```python
from build123d import *

# Parameters (mm, degrees)
BOSS_EXTRUDE1_DEPTH = 56.75
SKETCH2_W           = 5
SKETCH2_H           = 85
SKETCH2_R           = 1.5875
CUT_EXTRUDE1_DEPTH  = 2
SKETCH3_R           = 6.35
SKETCH3_R_2         = 1.5875
CUT_EXTRUDE2_DEPTH  = 3
CHAMFER1_SIZE       = 0.5
CUT_EXTRUDE3_DEPTH  = 5.5
CUT_EXTRUDE4_DEPTH  = 10


with BuildPart() as part:
    # Sketch1 → Boss-Extrude1 (new body, symmetric)
    with BuildSketch(Plane.XY):
        Polygon((0, 50), (0, -50), (7.5, -50), (7.5, -42.5), (2, -42.5), (2, 42.5), (7.5, 42.5), (7.5, 50), align=None)
    extrude(amount=BOSS_EXTRUDE1_DEPTH, both=True)

    # Sketch2 → Cut-Extrude1 (cut)
    with BuildSketch(Plane(origin=(2, 0, 0), x_dir=(0, 0, -1), z_dir=(1, 0, 0))):
        with Locations((-54.25, 0)):
            Rectangle(SKETCH2_W, SKETCH2_H)
        with Locations((54.25, 0)):
            Rectangle(SKETCH2_W, SKETCH2_H)
        with Locations((-47.75, 17.5)):
            Circle(SKETCH2_R)
        with Locations((-47.75, -17.5)):
            Circle(SKETCH2_R)
        with Locations((47.75, 17.5)):
            Circle(SKETCH2_R)
        with Locations((47.75, -17.5)):
            Circle(SKETCH2_R)
    extrude(amount=-CUT_EXTRUDE1_DEPTH, mode=Mode.SUBTRACT)

    # Sketch3 → Cut-Extrude2 (cut, through all)
    with BuildSketch(Plane(origin=(2, 0, 0), x_dir=(0, 0, -1), z_dir=(1, 0, 0))):
        Circle(SKETCH3_R)
        with Locations((39.75, 30.5)):
            Circle(SKETCH3_R_2)
        with Locations((39.75, -30.5)):
            Circle(SKETCH3_R_2)
        with BuildLine():
            Line((-29.899655804, -39.5), (29.899655804, -39.5))
            ThreePointArc((29.899655804, -39.5), (32.863003185, -37.464823364), (32.027336169, -33.968392001))
            Line((32.027336169, -33.968392001), (8.946350194, -13.129558949))
            ThreePointArc((8.946350194, -13.129558949), (7.399307524, -12.392275536), (5.701057458, -12.622220243))
            ThreePointArc((5.701057458, -12.622220243), (0, -13.85), (-5.701057458, -12.622220243))
            ThreePointArc((-5.701057458, -12.622220243), (-7.399307524, -12.392275536), (-8.946350194, -13.129558949))
            Line((-8.946350194, -13.129558949), (-32.027336169, -33.968392001))
            ThreePointArc((-32.027336169, -33.968392001), (-32.863003185, -37.464823364), (-29.899655804, -39.5))
        make_face()
        with BuildLine():
            Line((-43.75, -27.303546383), (-43.75, 27.303546383))
            ThreePointArc((-43.75, 27.303546383), (-41.864426198, 30.204926241), (-38.447319635, 29.660154382))
            Line((-38.447319635, 29.660154382), (-13.972366805, 7.562768399))
            ThreePointArc((-13.972366805, 7.562768399), (-13.081370721, 6.098851109), (-13.137175803, 4.386013216))
            ThreePointArc((-13.137175803, 4.386013216), (-13.85, 0), (-13.137175803, -4.386013216))
            ThreePointArc((-13.137175803, -4.386013216), (-13.081370721, -6.098851109), (-13.972366805, -7.562768399))
            Line((-13.972366805, -7.562768399), (-38.447319635, -29.660154382))
            ThreePointArc((-38.447319635, -29.660154382), (-41.864426198, -30.204926241), (-43.75, -27.303546383))
        make_face()
        with BuildLine():
            Line((-29.899655804, 39.5), (29.899655804, 39.5))
            ThreePointArc((29.899655804, 39.5), (32.863003185, 37.464823364), (32.027336169, 33.968392001))
            Line((32.027336169, 33.968392001), (8.946350194, 13.129558949))
            ThreePointArc((8.946350194, 13.129558949), (7.399307524, 12.392275536), (5.701057458, 12.622220243))
            ThreePointArc((5.701057458, 12.622220243), (0, 13.85), (-5.701057458, 12.622220243))
            ThreePointArc((-5.701057458, 12.622220243), (-7.399307524, 12.392275536), (-8.946350194, 13.129558949))
            Line((-8.946350194, 13.129558949), (-32.027336169, 33.968392001))
            ThreePointArc((-32.027336169, 33.968392001), (-32.863003185, 37.464823364), (-29.899655804, 39.5))
        make_face()
        with BuildLine():
            Line((43.75, -20.159375539), (43.75, 20.159375539))
            ThreePointArc((43.75, 20.159375539), (39.978852396, 25.962135255), (33.144639269, 24.872591538))
            Line((33.144639269, 24.872591538), (13.972366805, 7.562768399))
            ThreePointArc((13.972366805, 7.562768399), (13.081370721, 6.098851109), (13.137175803, 4.386013216))
            ThreePointArc((13.137175803, 4.386013216), (13.85, 0), (13.137175803, -4.386013216))
            ThreePointArc((13.137175803, -4.386013216), (13.081370721, -6.098851109), (13.972366805, -7.562768399))
            Line((13.972366805, -7.562768399), (33.144639269, -24.872591538))
            ThreePointArc((33.144639269, -24.872591538), (39.978852396, -25.962135255), (43.75, -20.159375539))
        make_face()
    extrude(amount=-CUT_EXTRUDE2_DEPTH, mode=Mode.SUBTRACT)

    # Chamfer1
    chamfer1_edges = [part.edges().sort_by_distance(p)[0] for p in [
        (0, -50, 0),
        (0, 50, 0),
    ]]
    chamfer(chamfer1_edges, length=CHAMFER1_SIZE)

    # Sketch4 → Cut-Extrude3 (cut)
    with BuildSketch(Plane(origin=(7.5, 0, 0), x_dir=(0, 0, -1), z_dir=(1, 0, 0))):
        with BuildLine():
            Line((43.575, -48), (-43.575, -48))
            ThreePointArc((-43.575, -48), (-45.82006403, -47.07006403), (-46.75, -44.825))
            Line((-46.75, -44.825), (-46.75, -43.5))
            ThreePointArc((-46.75, -43.5), (-47.042893219, -42.792893219), (-47.75, -42.5))
            Line((-47.75, -42.5), (47.75, -42.5))
            ThreePointArc((47.75, -42.5), (47.042893219, -42.792893219), (46.75, -43.5))
            Line((46.75, -43.5), (46.75, -44.825))
            ThreePointArc((46.75, -44.825), (45.82006403, -47.07006403), (43.575, -48))
        make_face()
        with BuildLine():
            Line((-46.75, 44.825), (-46.75, 43.5))
            ThreePointArc((-46.75, 43.5), (-47.042893219, 42.792893219), (-47.75, 42.5))
            Line((-47.75, 42.5), (47.75, 42.5))
            ThreePointArc((47.75, 42.5), (47.042893219, 42.792893219), (46.75, 43.5))
            Line((46.75, 43.5), (46.75, 44.825))
            ThreePointArc((46.75, 44.825), (45.82006403, 47.07006403), (43.575, 48))
            Line((43.575, 48), (-43.575, 48))
            ThreePointArc((-43.575, 48), (-45.82006403, 47.07006403), (-46.75, 44.825))
        make_face()
    extrude(amount=-CUT_EXTRUDE3_DEPTH, mode=Mode.SUBTRACT)

    # Sketch5 → Cut-Extrude4 (cut)
    with BuildSketch(Plane.ZY):
        with BuildLine():
            ThreePointArc((-51.75, 27.820508076), (-51.409258263, 30.408698527), (-50.410254038, 32.820508076))
            Line((-50.410254038, 32.820508076), (-48.285898385, 36.5))
            ThreePointArc((-48.285898385, 36.5), (-48.285898385, 40.5), (-51.75, 42.5))
            Line((-51.75, 42.5), (-51.75, 27.820508076))
        make_face()
        with BuildLine():
            ThreePointArc((-50.410254038, -32.820508076), (-51.409258263, -30.408698527), (-51.75, -27.820508076))
            Line((-51.75, -27.820508076), (-51.75, -42.5))
            ThreePointArc((-51.75, -42.5), (-48.285898385, -40.5), (-48.285898385, -36.5))
            Line((-48.285898385, -36.5), (-50.410254038, -32.820508076))
        make_face()
    cut_extrude4 = extrude(amount=-CUT_EXTRUDE4_DEPTH, mode=Mode.SUBTRACT)

    # Mirror1: Cut-Extrude4 across plane
    add(cut_extrude4.mirror(Plane.XY), mode=Mode.SUBTRACT)


solid = part.part
```
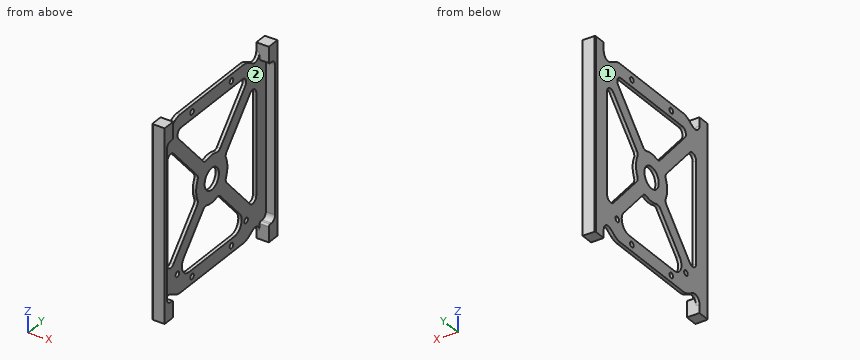
Geometry check sheet. Reference: the model listing, model coordinates, mm. Face numbers are marked on the shaded views. Give positions to 0.01 mm unless a question says otherwise; leave off trailing zeros. Write each loop counter-clockwise with the first axis right and the second up, starting at its lowest first coordinate (ties: lowest second). Pieces come first, ordered by that corner, then holes. Notation, with made-up numbers: (43.5, 21) - (59.5, 21) arc R18 cw to (59.5, 26) - close; hole circle Ø1 at (-17.75, 86.5). An arc over 180 degrees is marked (long way). Use a Markdown table: item, result.
Q1. Thickness scan on L1, parallel to Y at x = 2.25, z = 20.5; L2, parallel to Z at x = 1.25, y = 4.5; L3, parallel to Z at x = 0.5, y = 3. Record the ranges inside material, lowest first. Write a range as [from, to].
Computed:
| item | result |
|---|---|
| L1 | y = [-50, -48], [48, 50] |
| L2 | z = [-51.75, -43.75], [-13.1, -4.48], [4.48, 13.1], [43.75, 51.75] |
| L3 | z = [-51.75, -43.75], [-13.52, -5.6], [5.6, 13.52], [43.75, 51.75] |
Q2. Section check B-B, the plane x = 4.25. Enter the section's corners in (y, z) (3 decimals), then the cut area to 3 significant figures.
Computed:
| item | result |
|---|---|
| outline | (-50, -56.75) - (-42.5, -56.75) - (-42.5, -47.75) arc R1 ccw to (-43.5, -46.75) - (-44.825, -46.75) arc R3.175 cw to (-48, -43.575) - (-48, 43.575) arc R3.175 cw to (-44.825, 46.75) - (-43.5, 46.75) arc R1 ccw to (-42.5, 47.75) - (-42.5, 56.75) - (-50, 56.75) - close; (42.5, -56.75) - (50, -56.75) - (50, 56.75) - (42.5, 56.75) - (42.5, 47.75) arc R1 ccw to (43.5, 46.75) - (44.825, 46.75) arc R3.175 cw to (48, 43.575) - (48, -43.575) arc R3.175 cw to (44.825, -46.75) - (43.5, -46.75) arc R1 ccw to (42.5, -47.75) - close |
| area | 682 mm² |
Q3. Go/stop test with flat-tipped pins: P1, Ø0.6, axis at x = 1.5, y = -13, coming from the +Z side; P2, Ø1.6, axis at x = 1, y = -3.5, coming from the -Z side; P3, Ø3.5, axis at y = -17.5, z = 47.75, coming from the +X side. Record where each tip stops, or that it passes through.
Computed:
| item | result |
|---|---|
| P1 | stops at z = 51.75 |
| P2 | stops at z = -51.75 |
| P3 | stops at x = 2 |
Q4. Section check D-D, the plane y = -17.5. Enter the section's corners in (x, z), then the cut area to 3 significant figures.
Computed:
| item | result |
|---|---|
| outline | (0, -51.75) - (2, -51.75) - (2, -49.34) - (0, -49.34) - close; (0, -46.16) - (2, -46.16) - (2, -43.75) - (0, -43.75) - close; (0, -24.98) - (2, -24.98) - (2, -13.79) - (0, -13.79) - close; (0, 13.79) - (2, 13.79) - (2, 24.98) - (0, 24.98) - close; (0, 43.75) - (2, 43.75) - (2, 46.16) - (0, 46.16) - close; (0, 49.34) - (2, 49.34) - (2, 51.75) - (0, 51.75) - close |
| area | 64.1 mm² |
Q5. Draft check along Z on the marked faces 1 and 2. Enter one of: pulls with the +Z half, pulls with the -Z half, needs draft (parallel to the pull), parting line crosses it, or undercut.
Computed:
| item | result |
|---|---|
| face 1 | needs draft |
| face 2 | undercut |
Q6. Section check C-C, the plane z = 34.5. Enter the section's corners in (x, y), then the cut area to 3 significant figures.
Computed:
| item | result |
|---|---|
| outline | (0, -49.5) - (0.5, -50) - (7.5, -50) - (7.5, -48) - (2, -48) - (2, -26.1) - (0, -26.1) - close; (0, 26.1) - (2, 26.1) - (2, 48) - (7.5, 48) - (7.5, 50) - (0.5, 50) - (0, 49.5) - close |
| area | 117 mm² |
Q7. Section check A-A, the plane z = 0. Enter the section's corners in (x, y).
Computed:
| item | result |
|---|---|
| outline | (0, -49.5) - (0.5, -50) - (7.5, -50) - (7.5, -48) - (2, -48) - (2, -39.5) - (0, -39.5) - close; (0, -13.85) - (2, -13.85) - (2, -6.35) - (0, -6.35) - close; (0, 6.35) - (2, 6.35) - (2, 13.85) - (0, 13.85) - close; (0, 39.5) - (2, 39.5) - (2, 48) - (7.5, 48) - (7.5, 50) - (0.5, 50) - (0, 49.5) - close |
